Autodesk Inventor part; units mm, degrees
ref_plane "YZ Plane" through (0, 0, 0) normal (1, 0, 0) x (0, 1, 0)
ref_plane "XZ Plane" through (0, 0, 0) normal (0, 1, 0) x (-1, 0, 0)
ref_plane "XY Plane" through (0, 0, 0) normal (0, 0, 1) x (1, 0, 0)
sketch "Sketch1" plane through (0, 0, 0) normal (0, 0, 1) x (1, 0, 0)
  line L0 (-325, 250) -> (325, 250)
  line L1 (375, 200) -> (375, -200)
  line L2 (325, -250) -> (-325, -250)
  line L3 (-375, -200) -> (-375, 200)
  line L4 (-375, 250) -> (375, -250) construction
  line L5 (375, 250) -> (-375, -250) construction
  arc A0 (-325, 250) -> (-375, 200) centre (-325, 200) ccw
  arc A1 (-375, -200) -> (-325, -250) centre (-325, -200) ccw
  arc A2 (375, 200) -> (325, 250) centre (325, 200) ccw
  arc A3 (325, -250) -> (375, -200) centre (325, -200) ccw
  point P0 (0, 0)
  dimension "d0" = 750
  dimension "d1" = 500
  dimension "d2" = 50
extrude "Extrusion1" add sketch "Sketch1" along normal blind 2
sketch "Sketch2" plane through (0, 0, 2) normal (0, 0, 1) x (1, 0, 0)
  line L0 (-340, 220) -> (340, 220)
  line L1 (340, 220) -> (340, -220)
  line L2 (340, -220) -> (-340, -220)
  line L3 (-340, -220) -> (-340, 220)
  line L4 (-340, 220) -> (340, -220) construction
  line L5 (340, 220) -> (-340, -220) construction
  line L6 (300, 180) -> (-300, 180)
  line L7 (-300, 180) -> (-300, -180)
  line L8 (-300, -180) -> (300, -180)
  line L9 (300, -180) -> (300, 180)
  line L10 (300, 180) -> (180, 180)
  line L11 (180, 180) -> (180, -180)
  line L12 (180, -180) -> (300, -180)
  line L13 (300, -180) -> (300, 180)
  line L14 (-300, 180) -> (-180, 180)
  line L15 (-180, 180) -> (-180, -180)
  line L16 (-180, -180) -> (-300, -180)
  line L17 (-300, -180) -> (-300, 180)
  line L18 (-140, -180) -> (140, -180)
  line L19 (140, -180) -> (140, 180)
  line L20 (140, 180) -> (-140, 180)
  line L21 (-140, 180) -> (-140, -180)
  line L22 (-140, -180) -> (140, 180) construction
  line L23 (140, -180) -> (-140, 180) construction
  line L24 (-150, 180) -> (-150, -180)
  line L25 (-170, 180) -> (-170, -180)
  line L26 (170, 180) -> (170, -180)
  line L27 (150, 180) -> (150, -180)
  line L28 (330, 210) -> (-330, 210)
  line L29 (-330, 210) -> (-330, -210)
  line L30 (-330, -210) -> (330, -210)
  line L31 (330, -210) -> (330, 210)
  line L32 (-310, 190) -> (310, 190)
  line L33 (310, 190) -> (310, -190)
  line L34 (310, -190) -> (-310, -190)
  line L35 (-310, -190) -> (-310, 190)
  circle A0 centre (0, -190) radius 2.75
  circle A1 centre (0, -210) radius 2.75
  circle A2 centre (0, 190) radius 2.75
  circle A3 centre (0, 210) radius 2.75
  circle A4 centre (-213.335, 210) radius 2.75
  circle A5 centre (-213.335, 190) radius 2.75
  circle A6 centre (-310, 120) radius 2.75
  circle A7 centre (-330, 120) radius 2.75
  circle A8 centre (-330, -120) radius 2.75
  circle A9 centre (-310, -120) radius 2.75
  circle A10 centre (-213.335, -190) radius 2.75
  circle A11 centre (-213.335, -210) radius 2.75
  circle A12 centre (213.335, 190) radius 2.75
  circle A13 centre (213.335, 210) radius 2.75
  circle A14 centre (213.335, -190) radius 2.75
  circle A15 centre (213.335, -210) radius 2.75
  circle A16 centre (310, 120) radius 2.75
  circle A17 centre (330, 120) radius 2.75
  circle A18 centre (310, -120) radius 2.75
  circle A19 centre (330, -120) radius 2.75
  circle A20 centre (-170, 120) radius 2.75
  circle A21 centre (-150, 120) radius 2.75
  circle A22 centre (150, 120) radius 2.75
  circle A23 centre (170, 120) radius 2.75
  circle A24 centre (-170, -120) radius 2.75
  circle A25 centre (-150, -120) radius 2.75
  circle A26 centre (150, -120) radius 2.75
  circle A27 centre (170, -120) radius 2.75
  line L36 (-125, 172.5) -> (125, 172.5)
  line L37 (125, 172.5) -> (125, 97.5)
  line L38 (125, 97.5) -> (-125, 97.5)
  line L39 (-125, 97.5) -> (-125, 172.5)
  line L40 (-125, -97.5) -> (125, -97.5)
  line L41 (125, -97.5) -> (125, -172.5)
  line L42 (125, -172.5) -> (-125, -172.5)
  line L43 (-125, -172.5) -> (-125, -97.5)
  circle A28 centre (77, 24) radius 5.05
  circle A29 centre (-77, 24) radius 5.05
  circle A30 centre (77, -24) radius 5.05
  circle A31 centre (-77, -24) radius 5.05
  point P0 (0, 0)
  dimension "d5" = 680
  dimension "d6" = 440
  dimension "d17" = 280
  dimension "d18" = 10
  dimension "d19" = 10
  dimension "d20" = 10
  dimension "d21" = 10
  dimension "d22" = 360
  dimension "d23" = 180
  dimension "d24" = 300
  dimension "d25" = 40
  dimension "d26" = 10
  dimension "d27" = 20
  dimension "d28" = 5.5
  dimension "d29" = 5.5
  dimension "d30" = 5.5
  dimension "d31" = 5.5
  dimension "d32" = 5.5
  dimension "d33" = 5.5
  dimension "d34" = 5.5
  dimension "d35" = 5.5
  dimension "d36" = 5.5
  dimension "d37" = 5.5
  dimension "d38" = 5.5
  dimension "d39" = 5.5
  dimension "d40" = 5.5
  dimension "d41" = 5.5
  dimension "d42" = 5.5
  dimension "d43" = 5.5
  dimension "d44" = 5.5
  dimension "d45" = 5.5
  dimension "d46" = 5.5
  dimension "d47" = 5.5
  dimension "d48" = 233.33
  dimension "d49" = 193.33
  dimension "d50" = 193.33
  dimension "d51" = 233.33
  dimension "d52" = 233.33
  dimension "d53" = 193.33
  dimension "d54" = 233.33
  dimension "d55" = 193.33
  dimension "d56" = 60
  dimension "d57" = 60
  dimension "d58" = 60
  dimension "d59" = 60
  dimension "d60" = 60
  dimension "d61" = 60
  dimension "d62" = 60
  dimension "d63" = 60
  dimension "d64" = 5.5
  dimension "d65" = 5.5
  dimension "d66" = 5.5
  dimension "d67" = 5.5
  dimension "d68" = 5.5
  dimension "d69" = 5.5
  dimension "d70" = 5.5
  dimension "d71" = 5.5
  dimension "d72" = 60
  dimension "d73" = 60
  dimension "d74" = 60
  dimension "d75" = 60
  dimension "d76" = 60
  dimension "d77" = 60
  dimension "d78" = 60
extrude "Extrusion2" cut sketch "Sketch2" against normal through all contours A23 L26 | L26 A23 | A22 L27 | L27 A22 | A27 L26 | L26 A27 | A26 L27 | L27 A26 | A21 L24 | L24 A21 | A20 L25 | L25 A20 | A25 L24 | L24 A25 | A24 L25 | L25 A24 | A13 L28 | L28 A13 | A17 L31 | L31 A17 | A3 L28 | L28 A3 | A19 L31 | L31 A19 | A4 L28 | L28 A4 | A15 L30 | L30 A15 | A7 L29 | L29 A7 | A1 L30 | L30 A1 | A8 L29 | L29 A8 | A11 L30 | L30 A11 | A12 L32 | L32 A12 | A16 L33 | L33 A16 | A2 L32 | L32 A2 | A18 L33 | L33 A18 | A5 L32 | L32 A5 | A14 L34 | L34 A14 | A6 L35 | L35 A6 | A0 L34 | L34 A0 | A9 L35 | L35 A9 | A10 L34 | L34 A10 | L36 L37 L38 L39 | L40 L41 L42 L43 | A28 | A29 | A30 | A31
sketch "Sketch4" plane through (0, 0, 2) normal (0, 0, 1) x (1, 0, 0)
  line L0 (-276.0768, 250) -> (273.9232, 250)
  line L1 (-140, 250) -> (-125, 250)
  line L2 (-125, -250) -> (-140, -250)
  line L3 (125, 250) -> (140, 250)
  line L4 (140, -250) -> (125, -250)
  line L5 (-375, -150.5131) -> (-375, 149.4869)
  line L6 (375, 90) -> (375, 75)
  line L7 (-375, 75) -> (-375, 90)
  line L8 (375, 149.4869) -> (375, -150.5131)
  line L9 (375, -75) -> (375, -90)
  line L10 (273.9232, -250) -> (-276.0768, -250)
  line L11 (125, 232.5) -> (125, 250)
  line L12 (140, 250) -> (140, 232.5)
  line L13 (-125, 250) -> (-125, 232.5)
  line L14 (-140, 232.5) -> (-140, 250)
  line L15 (-375, 90) -> (-357.5, 90)
  line L16 (-357.5, 75) -> (-375, 75)
  line L17 (-375, -75) -> (-357.5, -75)
  line L18 (-357.5, -90) -> (-376.0768, -90)
  line L19 (-140, -250) -> (-140, -232.5)
  line L20 (-125, -232.5) -> (-125, -250)
  line L21 (140, -232.5) -> (140, -250)
  line L22 (125, -250) -> (125, -232.5)
  line L23 (357.5, -75) -> (375, -75)
  line L24 (375, -90) -> (357.5, -90)
  line L25 (357.5, 90) -> (375, 90)
  line L26 (375, 75) -> (357.5, 75)
  arc A0 (-140, 232.5) -> (-125, 232.5) centre (-132.5, 232.5) ccw
  arc A1 (125, 232.5) -> (140, 232.5) centre (132.5, 232.5) ccw
  arc A2 (-357.5, 75) -> (-357.5, 90) centre (-357.5, 82.5) ccw
  arc A3 (-357.5, -90) -> (-357.5, -75) centre (-357.5, -82.5) ccw
  arc A4 (-125, -232.5) -> (-140, -232.5) centre (-132.5, -232.5) ccw
  arc A5 (140, -232.5) -> (125, -232.5) centre (132.5, -232.5) ccw
  arc A6 (357.5, -75) -> (357.5, -90) centre (357.5, -82.5) ccw
  arc A7 (357.5, 90) -> (357.5, 75) centre (357.5, 82.5) ccw
  circle A8 centre (132.5, 232.5) radius 2.5
  circle A9 centre (-132.5, 232.5) radius 2.5
  circle A10 centre (-357.5, 82.5) radius 2.5
  circle A11 centre (-357.5, -82.5) radius 2.5
  circle A12 centre (-132.5, -232.5) radius 2.5
  circle A13 centre (132.5, -232.5) radius 2.5
  circle A14 centre (357.5, -82.5) radius 2.5
  circle A15 centre (357.5, 82.5) radius 2.5
  line L27 (-375, 200) -> (-375, -200)
  line L28 (325, 250) -> (-325, 250)
  point P0 (0, 0)
  point P1 (-132.5, -250)
  point P2 (132.5, -250)
  point P3 (125, 236.9869)
  point P4 (-140, 236.9869)
  point P5 (-125, 236.9869)
  point P6 (140, 236.9869)
  point P7 (-363.5768, 75)
  point P8 (373.8194, -75)
  point P9 (361.4232, 75)
  point P10 (361.4232, -90)
  point P11 (125, -238.0131)
  point P12 (-140, -238.0131)
  point P13 (-132.5, 225)
  point P14 (375, 82.5)
  point P15 (350, 82.5)
  dimension "d101" = 750
  dimension "d102" = 15
  dimension "d103" = 0
  dimension "d104" = 250
  dimension "d105" = 235
  dimension "d106" = 15
  dimension "d107" = 15
  dimension "d108" = 15
  dimension "d109" = 150
  dimension "d110" = 160
  dimension "d111" = 15
  dimension "d113" = 160
  dimension "d114" = 15
  dimension "d115" = 15
  dimension "d116" = 250
  dimension "d117" = 250
  dimension "d118" = 15
  dimension "d119" = 5
  dimension "d120" = 5
  dimension "d121" = 5
  dimension "d122" = 5
  dimension "d123" = 5
  dimension "d124" = 5
  dimension "d125" = 5
  dimension "d126" = 5
  dimension "d127" = 17.5
  dimension "d128" = 5
  dimension "d129" = 750
  dimension "d131" = 500
  dimension "d132" = 0
  dimension "d133" = 0
  dimension "d134" = 17.5
  dimension "d135" = 17.5
  dimension "d136" = 7.5
  dimension "d137" = 17.5
  dimension "d138" = 17.5
  dimension "d139" = 17.5
  dimension "d140" = 17.5
  dimension "d141" = 25
  dimension "d142" = 150
hole "Hole2" at (-357.5, 82.5, 2) at (-357.5, -82.5, 2) at (-132.5, -232.5, 2) at (132.5, -232.5, 2) at (357.5, -82.5, 2) at (357.5, 82.5, 2) at (132.5, 232.5, 2) at (-132.5, 232.5, 2) direction (0, 0, -1) diameter 5 end through all
equation "\"BendRadius\" = Thickness"
equation "\"BendReliefWidth\" = Thickness"
equation "\"BendReliefDepth\" = 0.5 * Thickness"
equation "\"CornerReliefSize\" = 4 * Thickness"
equation "\"MinimumRemnant\" = 2 * Thickness"
equation "\"TransitionRadius\" = BendRadius"
equation "\"JacobiRadiusSize\" = BendRadius"
equation "\"GapSize\" = Thickness"
properties part number "plate2mm" material "Aluminum 6061"
Check sheet for the modelled part. Datum: model origin and axes. Units: mm. Round coordinates to 2 decimals unless told otherwise and drop trailing zeros. Order: outer loops, then holes, each group sorted by start corner. A loop starts at its lowest first (then second) coordinate and runs counter-clockwise, first axis right, second up. Notation, with made-up numbers: M -22,36.25 L -4,36.25 A17 cw -4,51.25 Z; hole C 8,-6.75 d9. An arc over 180 degrees is marked long. One line per item, written item: value. Start each with the question number.
1. Scan lines: line 1 along X through (y, z) = (-190, 0.9) (3 decimals); line 2 along Y through (x, z) = (77, 1.05); line 3 along Y through (x, z) = (-49.5, 1.1). Record each from-to range of solid material in increasing order.
2. Section check C-C on z = 0.45. Give the number of separate pieces and of enclosed holes in the cut face, and give its area (3 significant figures).
3. Section check B-B on x = 98.5. Enter the section's corners in (y, z).
4. Section check A-A on y = 152. Enter the section's corners in (x, z).
5. Gauge pin test, flat end, axial feed: P1, Ø4.5, axis at x = -170, y = 120, coming from the +Z side. Record the tip position at first contact, or that the pin passes through.
Results found:
1. line 1: -375 to -216.085, -210.585 to -2.75, 2.75 to 210.585, 216.085 to 375
1. line 2: -250 to -172.5, -97.5 to -29.05, -18.95 to 18.95, 29.05 to 97.5, 172.5 to 250
1. line 3: -250 to -172.5, -97.5 to 97.5, 172.5 to 250
2. separate pieces: 1
2. enclosed holes: 42
2. area: 334,000 mm^2
3. outline: M -250,0 L -172.5,0 L -172.5,2 L -250,2 Z; M -97.5,0 L 97.5,0 L 97.5,2 L -97.5,2 Z; M 172.5,0 L 250,0 L 250,2 L 172.5,2 Z
4. outline: M -375,0 L -125,0 L -125,2 L -375,2 Z; M 125,0 L 375,0 L 375,2 L 125,2 Z
5. P1: through
